The drawing under review shows one solid part. Ordinate dimensions are in mm from its lowest x, y, z. A direction names the side the tool comes from. Give positions to 0.01 mm unless a question says otherwise; leave off trailing zeros. Write each loop counter-clockwise with the first axis right and the second up, starting at its lowest first coordinate (ties: lowest second). Pieces come first, ordered by that corner, then holes. Notation, with made-up numbers: (10, -18.5) -> (69, -18.5) arc R20 cw to (69, 2.5) -> close; hole circle Ø6 at (45, 71). An arc over 180 degrees is marked (long way). Write item = value, one per line.
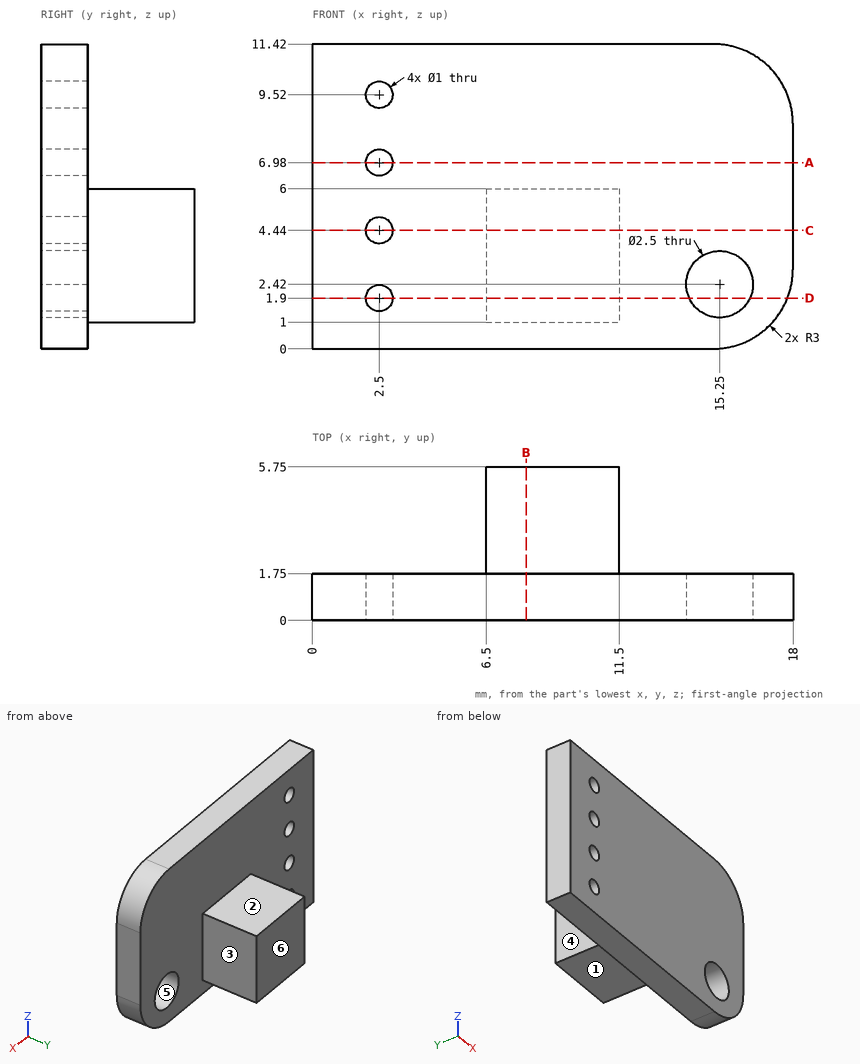
(1) Take a section at A-A (z = 6.98). Write out the cut boundary in (x, y), plus the area to 4 significant figures.
Answers below:
outline = (0, 0) -> (2, 0) -> (2, 1.75) -> (0, 1.75) -> close; (3, 0) -> (18, 0) -> (18, 1.75) -> (3, 1.75) -> close
area = 29.75 mm^2
(2) Take a section at C-C (z = 4.44). Write out the cut boundary in (x, y).
Answers below:
outline = (0, 0) -> (2, 0) -> (2, 1.75) -> (0, 1.75) -> close; (3, 0) -> (18, 0) -> (18, 1.75) -> (11.5, 1.75) -> (11.5, 5.75) -> (6.5, 5.75) -> (6.5, 1.75) -> (3, 1.75) -> close
(3) Take a section at B-B (x = 8). Write out the cut boundary in (y, z), plus the area to 3 significant figures.
Answers below:
outline = (0, 0) -> (1.75, 0) -> (1.75, 1) -> (5.75, 1) -> (5.75, 6) -> (1.75, 6) -> (1.75, 11.42) -> (0, 11.42) -> close
area = 40.0 mm^2
(4) Take a section at D-D (z = 1.9). Write out the cut boundary in (x, y), plus the area to 3 significant figures.
Answers below:
outline = (0, 0) -> (2, 0) -> (2, 1.75) -> (0, 1.75) -> close; (3, 0) -> (14.11, 0) -> (14.11, 1.75) -> (11.5, 1.75) -> (11.5, 5.75) -> (6.5, 5.75) -> (6.5, 1.75) -> (3, 1.75) -> close; (16.39, 0) -> (17.79, 0) -> (17.79, 1.75) -> (16.39, 1.75) -> close
area = 45.4 mm^2
(5) To check wall thickness, follow probe 1 along X at (y, z) = (0.9, 6.98); probe 2 along Y at (x, z) = (14, 3.5); probe 3 along X at (y, z) = (4.15, 3). State the ranges of each line that lie inside material, in increasing order.
Answers below:
probe_1 = 0 to 2, 3 to 18
probe_2 = 0 to 1.75
probe_3 = 6.5 to 11.5
(6) Tool access review of the marked faces 1, 2 and 3: name each direction out of +Z, -Z, +X, -X, +Y, -Y from which nothing blocks a thin tool from reaching the whole face with its end or side.
Answers below:
face_1 = -Z, +X, -X, +Y
face_2 = +Z, +X, -X, +Y
face_3 = +Z, -Z, +X, +Y
(7) The part is to be moulded in two halves that separate along X. For the marked faces 4, 5 and 6, say which applies: released by +X, released by -X, zero draft, split by the parting line, or undercut.
Answers below:
face_4 = released by -X
face_5 = undercut
face_6 = zero draft
(8) For pin 1 (3 mm diameter, centred on x = 15.25, z = 2.42, fed in from +Y); pin 2 (3 mm diameter, centred on x = 9, y = 4.5, fed in from -Z); pin 3 (2 mm diameter, centred on x = 9.5, y = 3, fed in from +Z), all flat-tipped, find the tip position at first contact; note any pin that passes through.
Answers below:
pin_1 = 1.75
pin_2 = 1
pin_3 = 6
